from build123d import *

# Parameters (mm, degrees)
EXTRUDE_1_DEPTH     = 5
SKETCH_19_W         = 5
SKETCH_19_H         = 18
EXTRUDE_2_DEPTH     = 1.5
FILLET_2_R          = 2
SKETCH_20_W         = 8
SKETCH_20_H         = 40
CUT_EXTRUDE_1_DEPTH = 36.961786675


with BuildPart() as part:
    # 扫描2: sweep along a path in 草图1
    with BuildLine(Plane.XY) as sweep_2_path:
        Line((11.886241035, 20.255064977), (10.916442642, 25.755064977))
        ThreePointArc((10.916442642, 25.755064977), (5.020643415, 30.27907084), (0, 24.8))
        Line((0, 24.8), (0, 0))
        Line((0, 0), (0, -2))
    # 草图13 → 扫描2 (sweep)
    with BuildSketch(Plane(origin=(0, -2, 0), x_dir=(1, 0, 0), z_dir=(0, 1, 0))):
        with BuildLine():
            Line((-1, -2.5), (1, -2.5))
            ThreePointArc((1, -2.5), (2.5, 0), (1, 2.5))
            Line((1, 2.5), (-1, 2.5))
            ThreePointArc((-1, 2.5), (-2.5, 0), (-1, -2.5))
        make_face()
    sweep(path=sweep_2_path.line)

    # 扫描4: sweep along a path in 草图15
    with BuildLine(Plane.XY) as sweep_4_path:
        Line((0, 0), (11, 0))
    # 草图16 → 扫描4 (sweep)
    with BuildSketch(Plane(origin=(11, 0, 0), x_dir=(0, 0, -1), z_dir=(1, 0, 0))):
        with BuildLine():
            Line((-2.5, -1), (-2.5, 1))
            ThreePointArc((-2.5, 1), (0, 2.5), (2.5, 1))
            Line((2.5, 1), (2.5, -1))
            ThreePointArc((2.5, -1), (0, -2.5), (-2.5, -1))
        make_face()
    sweep(path=sweep_4_path.line)

    # 草图17 → 凸台-拉伸1 (add)
    with BuildSketch(Plane(origin=(11, 0, 0), x_dir=(0, 0, -1), z_dir=(1, 0, 0))):
        with BuildLine():
            Line((-2.5, 1.555522876), (-2.5, -1.555522876))
            ThreePointArc((-2.5, -1.555522876), (0, -2.8), (2.5, -1.555522876))
            Line((2.5, -1.555522876), (2.5, 1.555522876))
            ThreePointArc((2.5, 1.555522876), (0, 2.8), (-2.5, 1.555522876))
        make_face()
    extrude(amount=-EXTRUDE_1_DEPTH)

    # 草图19 → 凸台-拉伸2 (add)
    with BuildSketch(Plane(origin=(1, 0, 0), x_dir=(0, 0, -1), z_dir=(1, 0, 0))):
        with Locations((0, 14)):
            Rectangle(SKETCH_19_W, SKETCH_19_H)
    extrude(amount=EXTRUDE_2_DEPTH)

    # 圆角2
    # the kernel refuses this fillet: 2 mm, written as the material it takes off along each edge
    with BuildSketch(Plane(origin=(17.795087554, 21.296954043, 2.5), x_dir=(0, 0, -1), z_dir=(-0.9848077530122092, -0.17364817766692373, 0))) as fillet_2_piece_1:
        with BuildLine():
            CenterArc((FILLET_2_R, -FILLET_2_R), FILLET_2_R, 90, 90)
            Line((0, -FILLET_2_R), (0, 0))
            Line((0, 0), (FILLET_2_R, 0))
        make_face()
    extrude(amount=12, mode=Mode.SUBTRACT)
    with BuildSketch(Plane(origin=(12.214510286, 20.312947703, 0), x_dir=(0.9423506208781959, 0.16616183974819204, -0.29045748456869663), z_dir=(0.2860447827236766, 0.05043741288507259, 0.9568878981667733))) as fillet_2_piece_2:
        with BuildLine():
            CenterArc((2.833333333 - FILLET_2_R, FILLET_2_R), FILLET_2_R, 270, 90)
            Line((2.833333333 - FILLET_2_R, 0), (2.833333333, 0))
            Line((2.833333333, 0), (2.833333333, FILLET_2_R))
        make_face()
    revolve(axis=Axis((12.214510286, 20.312947703, 0), (-0.173648177666923, 0.9848077530122094, 0)), revolution_arc=326.229306127, mode=Mode.SUBTRACT)
    with BuildSketch(Plane(origin=(5.977394517, 19.213175911, -2.5), x_dir=(-0.17364817766692373, 0.9848077530122092, 0), z_dir=(0.9848077530122092, 0.17364817766692373, 0))) as fillet_2_piece_3:
        with BuildLine():
            CenterArc((FILLET_2_R, FILLET_2_R), FILLET_2_R, 180, 90)
            Line((0, FILLET_2_R), (0, 0))
            Line((0, 0), (FILLET_2_R, 0))
        make_face()
    extrude(amount=12, mode=Mode.SUBTRACT)
    with BuildSketch(Plane(origin=(11, -6.555522876, 2.5), x_dir=(0, 0, -1), z_dir=(0, 1, 0))) as fillet_2_piece_4:
        with BuildLine():
            CenterArc((FILLET_2_R, FILLET_2_R), FILLET_2_R, 180, 90)
            Line((0, FILLET_2_R), (0, 0))
            Line((0, 0), (FILLET_2_R, 0))
        make_face()
    extrude(amount=13.111045751, mode=Mode.SUBTRACT)
    with BuildSketch(Plane(origin=(11, 6.555522876, -2.5), x_dir=(-1, 0, 0), z_dir=(0, -1, 0))) as fillet_2_piece_5:
        with BuildLine():
            CenterArc((FILLET_2_R, -FILLET_2_R), FILLET_2_R, 90, 90)
            Line((0, -FILLET_2_R), (0, 0))
            Line((0, 0), (FILLET_2_R, 0))
        make_face()
    extrude(amount=13.111045751, mode=Mode.SUBTRACT)
    with BuildSketch(Plane(origin=(11, -0.333333333, 0), x_dir=(0, -0.8131785022115455, -0.582014367125922), z_dir=(0, -0.582014367125922, 0.8131785022115455))) as fillet_2_piece_6:
        with BuildLine():
            CenterArc((3.133333333 - FILLET_2_R, -FILLET_2_R), FILLET_2_R, 0, 90)
            Line((3.133333333, -FILLET_2_R), (3.133333333, 0))
            Line((3.133333333, 0), (3.133333333 - FILLET_2_R, 0))
        make_face()
    revolve(axis=Axis((11, -0.333333333, 0), (1, 0, 0)), revolution_arc=288.815304863, mode=Mode.SUBTRACT)
    with BuildSketch(Plane(origin=(11, 0.333333333, 0), x_dir=(0, 0.8131785022115376, 0.5820143671259329), z_dir=(0, 0.5820143671259329, -0.8131785022115376))) as fillet_2_piece_7:
        with BuildLine():
            CenterArc((3.133333333 - FILLET_2_R, -FILLET_2_R), FILLET_2_R, 0, 90)
            Line((3.133333333 - FILLET_2_R, 0), (3.133333333, 0))
            Line((3.133333333, 0), (3.133333333, -FILLET_2_R))
        make_face()
    revolve(axis=Axis((11, 0.333333333, 0), (1, 0, 0)), revolution_arc=288.815304863, mode=Mode.SUBTRACT)
    with BuildSketch(Plane(origin=(11.557971784, 20.197182251, 0), x_dir=(-0.9423506208781961, -0.16616183974819207, 0.2904574845686964), z_dir=(-0.2860447827236764, -0.05043741288507257, -0.9568878981667737))) as fillet_2_piece_8:
        with BuildLine():
            CenterArc((2.833333333 - FILLET_2_R, FILLET_2_R), FILLET_2_R, 270, 90)
            Line((2.833333333, FILLET_2_R), (2.833333333, 0))
            Line((2.833333333, 0), (2.833333333 - FILLET_2_R, 0))
        make_face()
    revolve(axis=Axis((11.557971784, 20.197182251, 0), (-0.17364817766692306, 0.9848077530122095, 0)), revolution_arc=326.229306127, mode=Mode.SUBTRACT)

    # 草图20 → 切除-拉伸1 (cut, through all)
    with BuildSketch(Plane(origin=(-0.5, 0, 0), x_dir=(0, 0, -1), z_dir=(1, 0, 0))):
        with Locations((0, 16)):
            Rectangle(SKETCH_20_W, SKETCH_20_H)
    extrude(amount=-CUT_EXTRUDE_1_DEPTH, mode=Mode.SUBTRACT)


solid = part.part
Design review of the part built by this model. Coordinates are the model's own, in mm. A direction names the side the tool comes from. Coordinates: 2 decimals unless noted, no trailing zeros. Loops run counter-clockwise (first coordinate to the right, second up) from the corner with the lowest first, then second, coordinate; pieces in that order, holes last. Notation, with made-up numbers: M 22,25 L 45,25 A17 ccw 45,29 Z; hole C 88,-34.5 d7. An arc over 180 degrees is marked long. Use one line per item in the form item = value.
(1) Clearance check with flat-ended pins moving along their axes: P1, Ø3, axis at x = 0.5, z = -0.5, coming from the -Y side; P2, Ø1.7, axis at x = 2, z = -2, coming from the +Y side; P3, Ø0.5, axis at x = 2, z = 1.5, coming from the -Y side. State where each tip first meets the part, or that it passes through.
Return value:
P1 = -2.5
P2 = 31.87
P3 = -2.21
(2) Draft analysis for pull direction Y (two halves, no side actions). For faces 1 (the face through (11.755, 21.08, 2.126)), 2 (the face through (2, 23, 2)), 3 (the face through (2, 16, -2.5)), state which applies: pulls with the +Y half, pulls with the -Y half, needs draft (parallel to the pull), parting line crosses it, or undercut.
Return value:
face_1 = pulls with the -Y half
face_2 = undercut
face_3 = needs draft
(3) Consider section A-A (y = 15.5). Write out the cut boundary in (x, z), and give its area (3 significant figures).
Return value:
outline = M -0.5,-2.5 L 2.5,-2.5 L 2.5,2.5 L -0.5,2.5 Z
area = 15.0 mm2
(4) For faces 4 (the face through (10.13, -0.02, 2.15)), 5 (the face through (-0.3, -2, 0)), 6 (the face through (4.1, 2.5, 0)), 7 (the face through (11, 0, 0)), 8 (the face through (7.5, 2.8, 0)), list the 3-axis set-ups (+Z, -Z, +X, -X, +Y, -Y) from which the entire face can be reached by the end or side of a thin tool; tool diameter is ignored.
Return value:
face_4 = +Z, +X, -Y
face_5 = -X, -Y
face_6 = none
face_7 = +Z, -Z, +X, -Y
face_8 = +X
(5) For line 1 along X through (y, z) = (-0.5, 0.4); line 2 along X through (y, z) = (14, 0.45); line 3 along X through (y, z) = (27, 0.1), list the stretches that pass through material, from the lowest coordinate up. Write a range as from..to.
Return value:
line_1 = -0.5..11
line_2 = -0.5..2.5
line_3 = -0.5..3.46, 7.54..13.19
